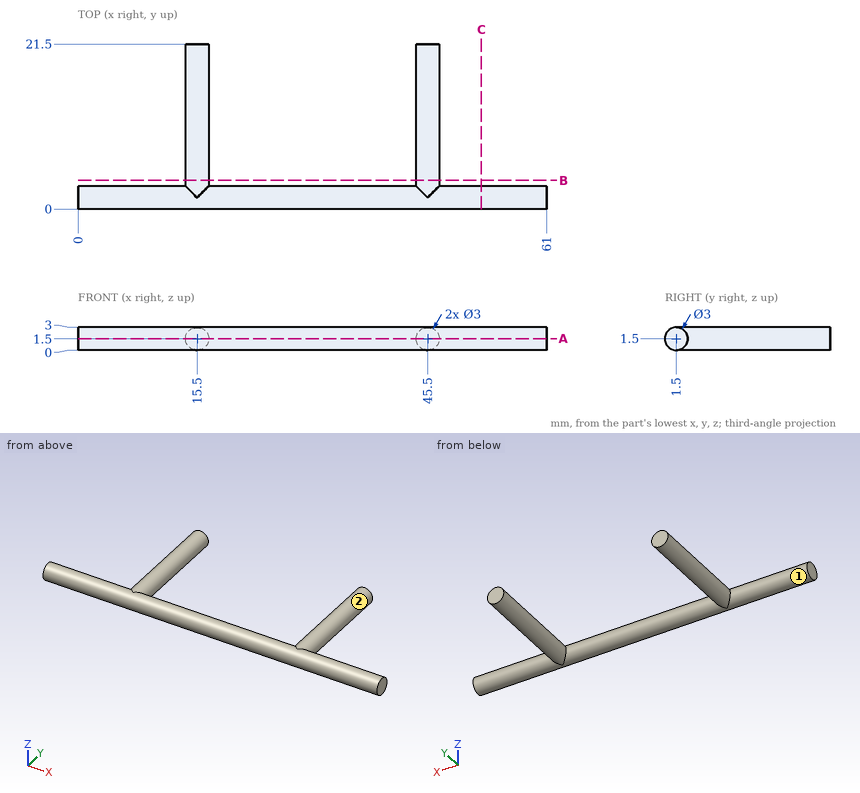
Here's the drawing with two shaded views (mm, measured from the low corner). I have some questions. A direction names the side the tool comes from. Coordinates: 2 decimals unless noted, no trailing zeros. Order: outer loops, then holes, each group sorted by start corner. A loop starts at its lowest first (then second) coordinate and runs counter-clockwise, first axis right, second up. Notation, with made-up numbers: (-5, 86.5) - (28, 86.5) arc R13 cw to (28, 104.5) - close; hole circle Ø6 at (-26.5, 63). An arc over 180 degrees is marked (long way). Use CSV: the item, a comma, the result in double quotes. Start each with the question number.
1. For the marked faces 1 and 2, which set-ups out of +Z, -Z, +X, -X, +Y, -Y let a thin tool reach every point of the face, with its end or its side?
2. Suppose I cut it at C-C on x = 52.5. List the corners of the cut face in (y, z) for me.
3. Please list where these lines run through material, in increasing order: line 1 (Y direction, x = 38.5, z = 1.3); line 2 (X direction, y = 17, z = 0.55); line 3 (X direction, y = 18, z = 0.95). Write a range as from..to.
4. Suppose I cut it at A-A on z = 1.5. List the corners of the cut face in (x, y) for me.
5. I'm going to push flat-ended pins straight in: pin 1 (1 mm diameter, centred on x = 36, y = 2.5, fed in from -Z); pin 2 (8 mm diameter, centred on x = 31, y = 10.5, fed in from +Z); pin 3 (1.5 mm diameter, centred on x = 40, z = 2, fed in from -Y). Where does each tip first touch, or does it pass through?
6. Suppose I cut it at B-B on y = 3.75. List the corners of the cut face in (x, z) for me.
Output:
1,face 1,"none"
1,face 2,"+Y"
2,outline,"circle Ø3 at (1.5, 1.5)"
3,line 1,"y = 0.01..2.99"
3,line 2,"x = 14.34..16.66, 44.34..46.66"
3,line 3,"x = 14.1..16.9, 44.1..46.9"
4,outline,"(0, 0) - (61, 0) - (61, 3) - (47, 3) - (47, 21.5) - (44, 21.5) - (44, 3) - (17, 3) - (17, 21.5) - (14, 21.5) - (14, 3) - (0, 3) - close"
5,pin 1,"stops at z = 0.09"
5,pin 2,"passes through"
5,pin 3,"stops at y = 0"
6,outline,"circle Ø3 at (15.5, 1.5); circle Ø3 at (45.5, 1.5)"
